CAD build for the part. Positions are in the model's coordinates, mm. Face numbers are marked on the shaded views. A direction names the side the tool comes from. Round coordinates to 2 decimals unless told otherwise and drop trailing zeros. Loops run counter-clockwise (first coordinate to the right, second up) from the corner with the lowest first, then second, coordinate; pieces in that order, holes last.
from build123d import *

# Parameters (mm, degrees)
F0_R          = 28.575
F0_R_2        = 7.9375
F1_DEPTH      = 12.7
F1_DEPTH_BACK = 12.7
F2_R          = 7.9375
F6_SIZE2      = 2.54
F6_SIZE       = 2.54
F7_R          = 1.5875
F8_W          = 4.7752
F8_H          = 10.3251
F9_DEPTH      = 15.4178
F9_DEPTH_BACK = 13.716


with BuildPart() as f1:
    # F0 (on Front) → F1 (new body, two sides)
    with BuildSketch(Plane.XZ) as f1_sk:
        Circle(F0_R)
        Circle(F0_R_2, mode=Mode.SUBTRACT)
    extrude(amount=F1_DEPTH)
    extrude(f1_sk.sketch, amount=-F1_DEPTH_BACK)

    # F2 (on Right) → F3 (revolve, cut)
    with BuildSketch(Plane.YZ):
        with Locations((0, 28.575016)):
            Circle(F2_R)
    revolve(axis=Axis((0, 66.637202, 0), (0, 1, 0)), mode=Mode.SUBTRACT)

    # F4 (on Right) → F5 (revolve, cut)
    with BuildSketch(Plane.YZ):
        Polygon((2.54, 19.05), (2.54, 12.7), (12.7, 12.7), (12.7, 25.4), align=None)
        Polygon((-12.7, 12.7), (-2.54, 12.7), (-2.54, 19.05), (-12.7, 25.4), align=None)
    revolve(axis=Axis((0, 24.1046, 0), (0, 1, 0)), mode=Mode.SUBTRACT)

    # F6
    f6_edges = [f1.edges().sort_by_distance(p)[0] for p in [
        (-28.575, 12.7, 0),
        (-28.575, -12.7, 0),
    ]]
    chamfer(f6_edges, length=F6_SIZE, length2=F6_SIZE2)

    # F7
    f7_edges = [f1.edges().sort_by_distance(p)[0] for p in [
        (0, 2.54, -12.7),
        (0, -2.54, -12.7),
    ]]
    fillet(f7_edges, radius=F7_R)

    # F8 (on Front) → F9 (cut, two sides)
    with BuildSketch(Plane.XZ) as f9_sk:
        with Locations((-0.350346, 5.16255)):
            Rectangle(F8_W, F8_H)
    extrude(amount=F9_DEPTH, mode=Mode.SUBTRACT)
    extrude(f9_sk.sketch, amount=-F9_DEPTH_BACK, mode=Mode.SUBTRACT)


solid = f1.part
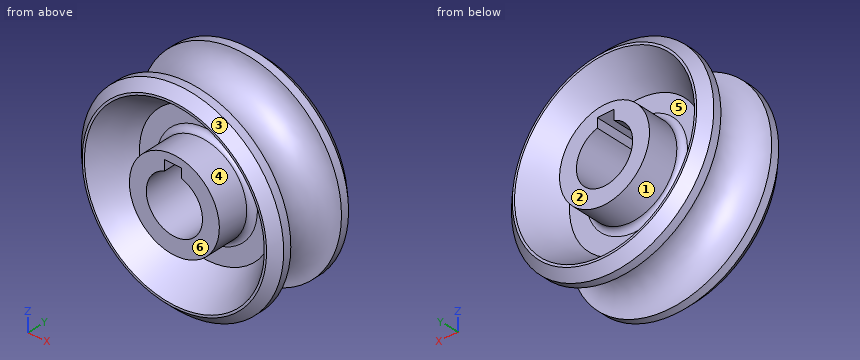
Item 1: Cut at B-B (y = -11). List the corners of the cut face in (x, z) (1 decimal).
Verdict:
outline: circle Ø55.5 at (0, 0); circle Ø25.4 at (0, 0); hole circle Ø48.7 at (0, 0); hole (-2.7, 7.5) arc R7.9 ccw (long way) to (2, 7.7) - (2, 10.3) - (-2.7, 10.3) - close
Item 2: Mould opens along Z. For the marked faces 1, 2 and 3 say: released by +Z, released by -Z, zero draft, split by the parting line, or undercut.
Verdict:
face 1: undercut
face 2: zero draft
face 3: split by the parting line
Item 3: 3-axis set-ups, long thin cutter, end or side, ignore diameter. For the marked faces 4, 5 and 6: which of +Z, -Z, +X, -X, +Y, -Y reach the whole face in a straight line?
Verdict:
face 4: -Y
face 5: +Y
face 6: +Z, -Z, +X, -X, -Y
Item 4: Wall check: L1, parallel to Z at x = 5.5, y = -6.5; L2, parallel to X at y = 9.5, z = 10; L3, parallel to X at y = 4, z = 0. Give the ranges that are in metal, low to high.
Verdict:
L1: z = -23.38 to -20.81, -11.45 to -5.72, 5.72 to 11.45, 20.81 to 23.38
L2: x = -26.77 to -21.16, -7.83 to -2.74, 2.04 to 7.83, 21.16 to 26.77
L3: x = -21.72 to -19.96, -12.71 to -7.94, 7.94 to 12.71, 19.96 to 21.72
Item 5: Flat gauge pins, fed straight in: P1, Ø8, axis at x = -17.5, y = 10, coming from the +Z side; P2, Ø1, axis at x = 22, y = 10, coming from the -Z side; P3, Ø8, axis at x = 11, y = 5, coming from the -Z side. Where does each tip first touch, or does it go through?
Verdict:
P1: stops at z = 25.18
P2: stops at z = -18.82
P3: stops at z = -27.35
Item 6: Cut at A-A (y = 7.25). List the corners of the cut face in (x, z) (1 decimal).
Verdict:
outline: circle Ø50.7 at (0, 0); circle Ø25.4 at (0, 0); hole circle Ø44 at (0, 0); hole (-2.7, 7.5) arc R7.9 ccw (long way) to (2, 7.7) - (2, 10.3) - (-2.7, 10.3) - close
